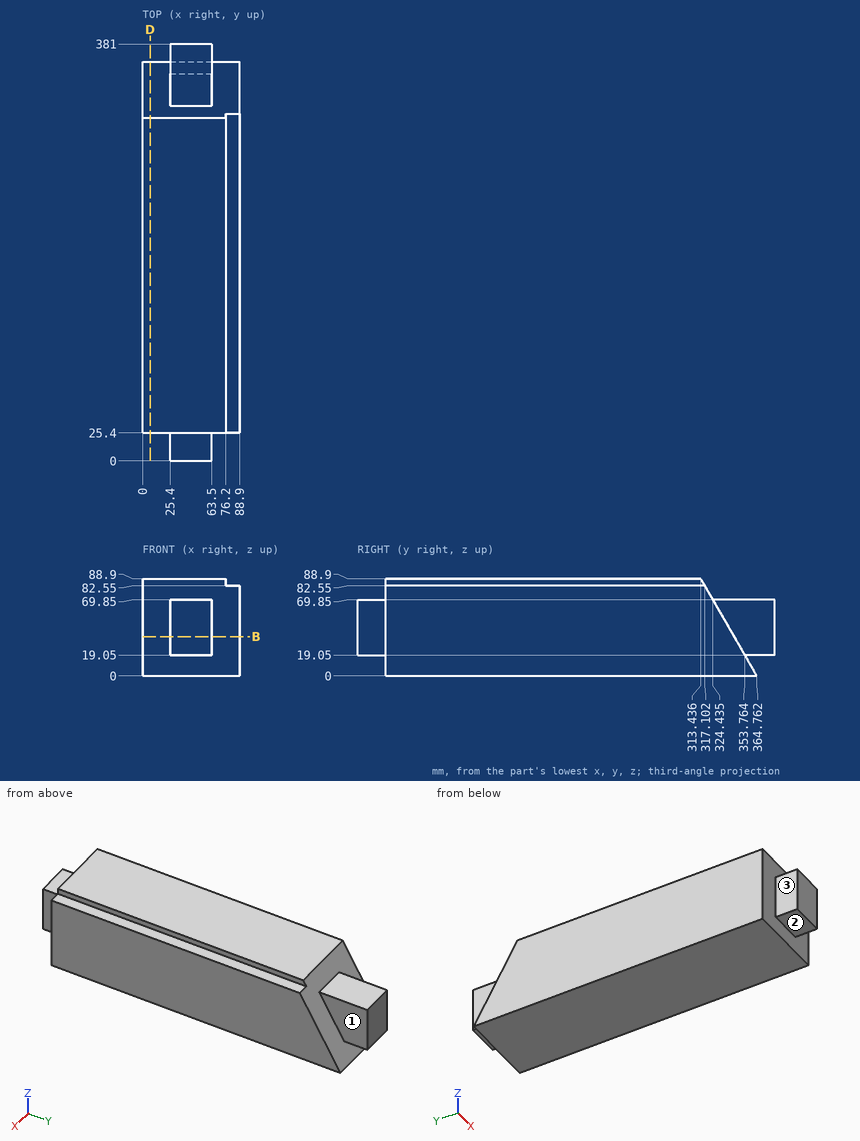
Can you work these out from the drawing? Everything is in mm from the part's minimum corner. A direction names the side the tool comes from. Coordinates: 2 decimals unless noted, no trailing zeros. Loops run counter-clockwise (first coordinate to the right, second up) from the corner with the lowest first, then second, coordinate; pieces in that order, holes last.
1) I need wall thicknesses on probe 1 along X at (y, z) = (197, 84); probe 2 along Z at (x, y) = (54.5, 352.5); probe 3 along Y at (x, z) = (80, 29). Which ranges of each line are inside material? Lowest first, please.
2) For pin 1 (7.5 mm diameter, centred on x = 48, y = 10, fed in from +Z); pin 2 (12.5 mm diameter, centred on y = 11.5, z = 55.5, fed in from +X); pin 3 (15 mm diameter, centred on y = 359, z = 47.5, fed in from -X), each with a flat end and sliding along its axis, tell me the tip position at first contact or that it passes through.
3) Imagine slicing it at D-D on x = 7. List the corners of the cut face in (y, z) for me, plus the area to 3 significant figures.
4) Which directions (+Z, -Z, +X, -X, +Y, -Y) give clear straight access to the entire face, cutting with the end or side of a thin tool? Please do the marked faces 1, 2 and 3.
5) Imagine slicing it at B-B on z = 36. List the corners of the cut face in (x, y) for me.
Completed:
1. probe 1: x = 0 to 76.2
1. probe 2: z = 0 to 69.85
1. probe 3: y = 25.4 to 348.02
2. pin 1: stops at z = 69.85
2. pin 2: stops at x = 63.5
2. pin 3: stops at x = 25.4
3. outline: (25.4, 0) - (364.76, 0) - (313.44, 88.9) - (25.4, 88.9) - close
3. area: 27,900 mm2
4. face 1: +Z, +X, +Y
4. face 2: -Z, +X, -X, -Y
4. face 3: +Z, -Z, -X, -Y
5. outline: (0, 25.4) - (25.4, 25.4) - (25.4, 0) - (63.5, 0) - (63.5, 25.4) - (88.9, 25.4) - (88.9, 343.98) - (63.5, 343.98) - (63.5, 381) - (25.4, 381) - (25.4, 343.98) - (0, 343.98) - close
